from build123d import *

# Parameters (mm, degrees)
BOSS_EXTRUDE1_DEPTH = 254
FILLET1_R           = 2.54


with BuildPart() as part:
    # Sketch1 → Boss-Extrude1 (new, symmetric)
    with BuildSketch(Plane(origin=(0, 0, 0), x_dir=(0, 0, -1), z_dir=(1, 0, 0))):
        with BuildLine():
            Line((0, 0), (271.296891492, 469.9))
            ThreePointArc((271.296891492, 469.9), (299.188027261, 497.791135768), (337.288027261, 508))
            Line((337.288027261, 508), (1143, 508))
            ThreePointArc((1143, 508), (1196.881536726, 485.681536726), (1219.2, 431.8))
            Line((1219.2, 431.8), (1219.2, 76.2))
            ThreePointArc((1219.2, 76.2), (1196.881536726, 22.318463274), (1143, 0))
            Line((1143, 0), (0, 0))
        make_face()
        with BuildLine():
            Line((337.288027261, 457.2), (1143, 457.2))
            ThreePointArc((1143, 457.2), (1160.960512242, 449.760512242), (1168.4, 431.8))
            Line((1168.4, 431.8), (1168.4, 76.2))
            ThreePointArc((1168.4, 76.2), (1160.960512242, 58.239487758), (1143, 50.8))
            Line((1143, 50.8), (87.988181024, 50.8))
            Line((87.988181024, 50.8), (315.290982004, 444.5))
            ThreePointArc((315.290982004, 444.5), (324.588027261, 453.797045256), (337.288027261, 457.2))
        make_face(mode=Mode.SUBTRACT)
    extrude(amount=BOSS_EXTRUDE1_DEPTH, both=True)

    # Fillet1
    fillet1_edges = [part.edges().sort_by_distance(p)[0] for p in [
        (0, 0, 0),
        (0, 50.8, -87.988181024),
    ]]
    fillet(fillet1_edges, radius=FILLET1_R)


solid = part.part
Input: part model. Units: mm. Frame: model coordinates. A direction names the side the tool comes from. Give positions to 0.01 mm unless a question says otherwise; leave off trailing zeros. Order: outer loops, then holes, each group sorted by start corner. A loop starts at its lowest first (then second) coordinate and runs counter-clockwise, first axis right, second up.
Q1. Section A-A on z = -849.5. Output: boundary loops of the cut face in (x, y), and give its area (3 significant figures).
Checked values:
outline: (-254, 0) - (254, 0) - (254, 50.8) - (-254, 50.8) - close; (-254, 457.2) - (254, 457.2) - (254, 508) - (-254, 508) - close
area: 51,600 mm2
Q2. Section D-D on y = 31. Output: boundary loops of the cut face in (x, z), and give its area (3 significant figures).
Checked values:
outline: (-254, -1204.35) - (254, -1204.35) - (254, -17.9) - (-254, -17.9) - close
area: 603,000 mm2
Q3. Section C-C on y = 254. Output: boundary loops of the cut face in (x, z).
Checked values:
outline: (-254, -1219.2) - (254, -1219.2) - (254, -1168.4) - (-254, -1168.4) - close; (-254, -205.31) - (254, -205.31) - (254, -146.65) - (-254, -146.65) - close
Q4. Section B-B on x = 39.5. Output: boundary loops of the cut face in (y, z).
Checked values:
outline: (0, -1143) arc R76.2 ccw to (76.2, -1219.2) - (431.8, -1219.2) arc R76.2 ccw to (508, -1143) - (508, -337.29) arc R76.2 ccw to (469.9, -271.3) - (3.81, -2.2) arc R2.54 ccw to (0, -4.4) - close; hole (50.8, -1143) arc R25.4 ccw to (76.2, -1168.4) - (431.8, -1168.4) arc R25.4 ccw to (457.2, -1143) - (457.2, -337.29) arc R25.4 ccw to (444.5, -315.29) - (54.61, -90.19) arc R2.54 ccw to (50.8, -92.39) - close
Q5. Contact query for flat-ended pins moving along their axis: pin 1 Ø10 at (x, y) = (-148.5, 347.5) entering from +Z; pin 2 Ø2 at (x, z) = (168.5, -170.5) entering from +Y; pin 3 Ø3 at (x, y) = (-106, 389.5) entering from +Z. Output: stop coordinate, or through.
Checked values:
pin 1: stops at z = -197.74
pin 2: stops at y = 297.05
pin 3: stops at z = -224.01
Q6. Ray query, probe 1 along Y at (x, z) = (121, -623); probe 2 along Y at (x, z) = (156, -193.5); probe 3 along Z at (x, y) = (90.5, 338.5). Return the intervals inside material, ascending.
Checked values:
probe 1: y = 0 to 50.8, 457.2 to 508
probe 2: y = 0 to 50.8, 233.55 to 335.15
probe 3: z = -1219.2 to -1168.4, -254.09 to -195.43
Q7. Set-up query: faces 1 (the cylindrical face through (3.556, 453.703, -324.427)), 2 (the flat face through (-254, 48, -613)). Return all of +Z, -Z, +X, -X, +Y, -Y with unobstructed straight access to the full face (end or side cutting, diameter ignored); none if empty.
Checked values:
face 1: +X, -X
face 2: +Z, -Z, -X, +Y, -Y
Q8. Draft query along Y for faces 3 (the flat face through (4, 0, -582)), 4 (the flat face through (3.556, 246.826, -201.164)), 5 (the cylindrical face through (3.556, 486.271, -1196.286)), 6 (the flat face through (254, 48, -613)). Return one class per face: +Y half, -Y half, draft (parallel to the pull), parting line (faces both ways), or undercut.
Checked values:
face 3: -Y half
face 4: undercut
face 5: +Y half
face 6: draft
